```python
from build123d import *

# Parameters (mm, degrees)
SKETCH1_R           = 20
SKETCH1_R_2         = 2
SKETCH1_R_3         = 2.5
BOSS_EXTRUDE1_DEPTH = 2


with BuildPart() as part:
    # Sketch1 → Boss-Extrude1 (new body)
    with BuildSketch(Plane.XY):
        with BuildLine():
            Line((-50, -78), (50, -78))
            Line((50, -78), (31.774896218, 6.82685655))
            ThreePointArc((31.774896218, 6.82685655), (0, 32.5), (-31.774896218, 6.82685655))
            Line((-31.774896218, 6.82685655), (-50, -78))
        make_face()
        Circle(SKETCH1_R, mode=Mode.SUBTRACT)
        with Locations((0, 28)):
            Circle(SKETCH1_R_2, mode=Mode.SUBTRACT)
        with Locations((24.248711306, 14)):
            Circle(SKETCH1_R_2, mode=Mode.SUBTRACT)
        with Locations((24.248711306, -14)):
            Circle(SKETCH1_R_2, mode=Mode.SUBTRACT)
        with Locations((-24.248711306, -14)):
            Circle(SKETCH1_R_2, mode=Mode.SUBTRACT)
        with Locations((-24.248711306, 14)):
            Circle(SKETCH1_R_2, mode=Mode.SUBTRACT)
        with Locations((0, -68)):
            Circle(SKETCH1_R_3, mode=Mode.SUBTRACT)
        with Locations((23, -43)):
            Circle(SKETCH1_R_3, mode=Mode.SUBTRACT)
        with Locations((-23, -43)):
            Circle(SKETCH1_R_3, mode=Mode.SUBTRACT)
    extrude(amount=BOSS_EXTRUDE1_DEPTH)


solid = part.part
```
The model under review builds one solid part; all positions refer to its coordinate system, in mm. Give positions to 0.01 mm unless a question says otherwise; leave off trailing zeros. Write each loop counter-clockwise with the first axis right and the second up, starting at its lowest first coordinate (ties: lowest second). Pieces come first, ordered by that corner, then holes. Notation, with made-up numbers: (22.25, -7.5) - (51.25, -7.5) arc R17 ccw to (51.25, 13.5) - close; hole circle Ø1 at (6.25, 30). An arc over 180 degrees is marked (long way). Answer in a Markdown table with one row per item. Add a question column.
1. Draft analysis for pull direction X (two halves, no side actions). For faces 1 (the flat face through (-40.76, -34.99, 0.99)), 2 (the cylindrical face through (26.156, 14.601, 0.986)), 3 (the flat face through (-1, -34, 2)), state which applies: +X half, -X half, draft (parallel to the pull), parting line (faces both ways), or undercut.
2. We need section C-C on z = 1.7. State how many separate pieces and enclosed holes the cut face has, then the cut area to 3 significant figures.
3. We need section D-D on y = -43. Write out the cut boundary in (x, z), then the cut area to 3 significant figures.
4. We need section B-B on x = 0. Write out the cut boundary in (y, z), then the cut area to 3 significant figures.
5. Wall thickness on line 1 along Y through (x, z) = (0, 0.65); line 2 along Y through (x, z) = (-23, 0.7); line 3 along X through (y, z) = (-15.5, 1.75): over which ranges is each line inside the solid? List them lowest first. Write a range as [from, to].
6. We need section A-A on y = 28. Write out the cut boundary in (x, z), then the cut area to 3 significant figures.
7. Insertion check: P1, Ø1, axis at y = -22, z = 1.5, coming from the +X side. The pin has a flat end and moves straight along its axis. Give the tip position at first contact, or say it passes through.
Ans:
| question | item | result |
|---|---|---|
| 1 | face 1 | -X half |
| 1 | face 2 | undercut |
| 1 | face 3 | draft |
| 2 | separate pieces | 1 |
| 2 | enclosed holes | 9 |
| 2 | area | 6,780 mm^2 |
| 3 | outline | (-42.48, 0) - (-25.5, 0) - (-25.5, 2) - (-42.48, 2) - close; (-20.5, 0) - (20.5, 0) - (20.5, 2) - (-20.5, 2) - close; (25.5, 0) - (42.48, 0) - (42.48, 2) - (25.5, 2) - close |
| 3 | area | 150 mm^2 |
| 4 | outline | (-78, 0) - (-70.5, 0) - (-70.5, 2) - (-78, 2) - close; (-65.5, 0) - (-20, 0) - (-20, 2) - (-65.5, 2) - close; (20, 0) - (26, 0) - (26, 2) - (20, 2) - close; (30, 0) - (32.5, 0) - (32.5, 2) - (30, 2) - close |
| 4 | area | 123 mm^2 |
| 5 | line 1 | y = [-78, -70.5], [-65.5, -20], [20, 26], [30, 32.5] |
| 5 | line 2 | y = [-78, -45.5], [-40.5, -15.56], [-12.44, 12.44], [15.56, 22.96] |
| 5 | line 3 | x = [-36.57, -25.57], [-22.93, -12.64], [12.64, 22.93], [25.57, 36.57] |
| 6 | outline | (-16.5, 0) - (-2, 0) - (-2, 2) - (-16.5, 2) - close; (2, 0) - (16.5, 0) - (16.5, 2) - (2, 2) - close |
| 6 | area | 58.0 mm^2 |
| 7 | P1 | stops at x = 38.08 |
